from build123d import *

# Parameters (mm, degrees)
SKETCH1_W           = 148
SKETCH1_H           = 62
BOSS_EXTRUDE1_DEPTH = 15
SKETCH2_R           = 2.25
CUT_EXTRUDE1_DEPTH  = 35
SKETCH3_R           = 2.25
CUT_EXTRUDE2_DEPTH  = 25
SKETCH4_W           = 22
SKETCH4_H           = 5
BOSS_EXTRUDE2_DEPTH = 26
SKETCH5_W           = 22
SKETCH5_H           = 5
BOSS_EXTRUDE3_DEPTH = 26
SKETCH6_W           = 20
SKETCH6_H           = 42
BOSS_EXTRUDE4_DEPTH = 15
SKETCH7_W           = 20
SKETCH7_H           = 42
BOSS_EXTRUDE5_DEPTH = 15
SKETCH8_R           = 2.5
CUT_EXTRUDE3_DEPTH  = 25
SKETCH9_R           = 2.5
CUT_EXTRUDE4_DEPTH  = 25
CHAMFER3_SIZE       = 1
CHAMFER4_SIZE       = 1
CHAMFER5_SIZE       = 1
SKETCH10_W          = 27.530750263
SKETCH10_H          = 14.173658936
CUT_EXTRUDE5_DEPTH  = 60
SKETCH11_W          = 32.495188708
SKETCH11_H          = 15.919959855
CUT_EXTRUDE6_DEPTH  = 60
CHAMFER6_SIZE       = 1
CHAMFER7_SIZE       = 1


with BuildPart() as part:
    # Sketch1 → Boss-Extrude1 (new body)
    with BuildSketch(Plane(origin=(0, 0, 0), x_dir=(1, 0, 0), z_dir=(0, 1, 0))):
        with Locations((74, 31)):
            Rectangle(SKETCH1_W, SKETCH1_H)
    extrude(amount=BOSS_EXTRUDE1_DEPTH)

    # Sketch2 → Cut-Extrude1 (cut)
    with BuildSketch(Plane(origin=(0, 15, 0), x_dir=(1, 0, 0), z_dir=(0, 1, 0))):
        with Locations(Location((5, 4, 0), (0, 0, 270))):
            Circle(SKETCH2_R)
        with Locations(Location((20, 4, 0), (0, 0, 270))):
            Circle(SKETCH2_R)
        with Locations(Location((35, 4, 0), (0, 0, 270))):
            Circle(SKETCH2_R)
        with Locations(Location((5, 58, 0), (0, 0, 270))):
            Circle(SKETCH2_R)
        with Locations(Location((20, 58, 0), (0, 0, 270))):
            Circle(SKETCH2_R)
        with Locations(Location((35, 58, 0), (0, 0, 270))):
            Circle(SKETCH2_R)
    extrude(amount=-CUT_EXTRUDE1_DEPTH, mode=Mode.SUBTRACT)

    # Sketch3 → Cut-Extrude2 (cut)
    with BuildSketch(Plane(origin=(0, 15, 0), x_dir=(1, 0, 0), z_dir=(0, 1, 0))):
        with Locations(Location((143, 58, 0), (0, 0, 270))):
            Circle(SKETCH3_R)
        with Locations(Location((143, 4, 0), (0, 0, 270))):
            Circle(SKETCH3_R)
        with Locations(Location((128, 58, 0), (0, 0, 270))):
            Circle(SKETCH3_R)
        with Locations(Location((113, 58, 0), (0, 0, 270))):
            Circle(SKETCH3_R)
        with Locations(Location((128, 4, 0), (0, 0, 270))):
            Circle(SKETCH3_R)
        with Locations(Location((113, 4, 0), (0, 0, 270))):
            Circle(SKETCH3_R)
    extrude(amount=-CUT_EXTRUDE2_DEPTH, mode=Mode.SUBTRACT)

    # Sketch4 → Boss-Extrude2 (add)
    with BuildSketch(Plane(origin=(148, 0, 0), x_dir=(0, 0, -1), z_dir=(1, 0, 0))):
        with Locations((31, 2.5)):
            Rectangle(SKETCH4_W, SKETCH4_H)
    extrude(amount=BOSS_EXTRUDE2_DEPTH)

    # Sketch5 → Boss-Extrude3 (add)
    with BuildSketch(Plane.ZY):
        with Locations((-31, 2.5)):
            Rectangle(SKETCH5_W, SKETCH5_H)
    extrude(amount=BOSS_EXTRUDE3_DEPTH)

    # Sketch6 → Boss-Extrude4 (add)
    with BuildSketch(Plane(origin=(0, 15, 0), x_dir=(1, 0, 0), z_dir=(0, 1, 0))):
        with Locations((184, 31)):
            Rectangle(SKETCH6_W, SKETCH6_H)
    extrude(amount=-BOSS_EXTRUDE4_DEPTH)

    # Sketch7 → Boss-Extrude5 (add)
    with BuildSketch(Plane(origin=(0, 15, 0), x_dir=(1, 0, 0), z_dir=(0, 1, 0))):
        with Locations((-36, 31)):
            Rectangle(SKETCH7_W, SKETCH7_H)
    extrude(amount=-BOSS_EXTRUDE5_DEPTH)

    # Sketch8 → Cut-Extrude3 (cut)
    with BuildSketch(Plane(origin=(0, 15, 0), x_dir=(1, 0, 0), z_dir=(0, 1, 0))):
        with Locations(Location((-36, 46, 0), (0, 0, 270))):
            Circle(SKETCH8_R)
        with Locations(Location((-36, 15, 0), (0, 0, 270))):
            Circle(SKETCH8_R)
    extrude(amount=-CUT_EXTRUDE3_DEPTH, mode=Mode.SUBTRACT)

    # Sketch9 → Cut-Extrude4 (cut)
    with BuildSketch(Plane(origin=(0, 15, 0), x_dir=(1, 0, 0), z_dir=(0, 1, 0))):
        with Locations(Location((184, 46, 0), (0, 0, 270))):
            Circle(SKETCH9_R)
        with Locations(Location((184, 15, 0), (0, 0, 270))):
            Circle(SKETCH9_R)
    extrude(amount=-CUT_EXTRUDE4_DEPTH, mode=Mode.SUBTRACT)

    # Chamfer3
    chamfer3_edges = [part.edges().sort_by_distance(p)[0] for p in [
        (194, 15, -31),
        (-26, 15, -31),
        (-46, 15, -31),
        (161, 5, -20),
    ]]
    chamfer(chamfer3_edges, length=CHAMFER3_SIZE)

    # Chamfer4
    chamfer4_edges = [part.edges().sort_by_distance(p)[0] for p in [
        (-13, 5, -20),
        (-36, 15, -10),
        (-36, 15, -52),
        (183.5, 15, -10),
        (183.5, 15, -52),
        (161, 5, -42),
    ]]
    chamfer(chamfer4_edges, length=CHAMFER4_SIZE)

    # Chamfer5
    chamfer5_edges = [part.edges().sort_by_distance(p)[0] for p in [
        (-13, 5, -42),
        (174, 15, -31),
    ]]
    chamfer(chamfer5_edges, length=CHAMFER5_SIZE)

    # Sketch10 → Cut-Extrude5 (cut)
    with BuildSketch(Plane(origin=(0, 0, -52), x_dir=(-1, 0, 0), z_dir=(0, 0, -1))):
        with Locations((-183.765375132, 12.086829468)):
            Rectangle(SKETCH10_W, SKETCH10_H)
    extrude(amount=-CUT_EXTRUDE5_DEPTH, mode=Mode.SUBTRACT)

    # Sketch11 → Cut-Extrude6 (cut)
    with BuildSketch(Plane(origin=(0, 0, -52), x_dir=(-1, 0, 0), z_dir=(0, 0, -1))):
        with Locations((37.724079719, 12.959979928)):
            Rectangle(SKETCH11_W, SKETCH11_H)
    extrude(amount=-CUT_EXTRUDE6_DEPTH, mode=Mode.SUBTRACT)

    # Chamfer6
    chamfer6_edges = [part.edges().sort_by_distance(p)[0] for p in [
        (174, 5, -46.5),
        (194, 5, -31),
        (174, 5, -15.5),
        (-46, 5, -31),
        (-36, 5, -10),
        (-26, 5, -46.5),
    ]]
    chamfer(chamfer6_edges, length=CHAMFER6_SIZE)

    # Chamfer7
    chamfer7_edges = [part.edges().sort_by_distance(p)[0] for p in [
        (-36, 5, -52),
        (-26, 5, -16),
        (184, 5, -10),
        (184, 5, -52),
    ]]
    chamfer(chamfer7_edges, length=CHAMFER7_SIZE)


solid = part.part
Verification items for the finished model (mm, model axes). A direction names the side the tool comes from. Give positions to 0.01 mm unless a question says otherwise; leave off trailing zeros. Write each loop counter-clockwise with the first axis right and the second up, starting at its lowest first coordinate (ties: lowest second). Pieces come first, ordered by that corner, then holes.
(1) Material ranges on line 1 (Z direction, x = 143, y = 11); line 2 (X direction, y = 2.3, z = -15); line 3 (Z direction, x = 19, y = 1.5), recorded low to high.
(2) Cross-section at B-B (z = -46). Enter the section's corners in (x, y), plus the area to 3 significant figures.
(3) Mould release check, pull along Z, two halves, no side actions. Record for faces 1 (the face through (174, 2, -15)), 2 (the face through (37.23, 7.6, -4.29)), 3 (the face through (184, 2, -10)): +Z half, -Z half, draft (parallel to the pull), parting line (faces both ways), or undercut.
(4) Gauge pin test, flat ends, axial feed: pin 1 (4 mm diameter, centred on x = 5, z = -58, fed in from +Y); pin 2 (4.5 mm diameter, centred on x = -19.5, y = 2.5, fed in from -Z); pin 3 (6.5 mm diameter, centred on x = 184, z = -46, fed in from +Y); pin 4 (3 mm diameter, centred on y = 7, z = -49, fed in from +X). Record the tip position at first contact, or that the pin passes through.
(5) Cross-section at A-A (x = 128). Enter the section's corners in (y, z), plus the area to 3 significant figures.
(6) Cross-section at D-D (y = 10). State how many separate pieces and enclosed holes the cut face has, plus the area to 3 significant figures.
(7) Cross-section at C-C (z = -4). Enter the section's corners in (x, y).
(8) Access from +Z, -Z, +X, -X, +Y, -Y to the whole of each face (thin tool, end or side, straight path). Record for faces 4 (the face through (-13, 2, -42)), 5 (the face through (-27, 5, -31)), 6 (the face through (-26, 2, -15)).
Worked out:
1. line 1: z = -62 to -60.25, -55.75 to -6.25, -1.75 to 0
1. line 2: x = -46 to -38.5, -33.5 to -26, 0 to 148, 174 to 181.5, 186.5 to 194
1. line 3: z = -62 to -60.02, -55.98 to -6.02, -1.98 to 0
2. outline: (-46, 0) - (-38.5, 0) - (-38.5, 5) - (-45, 5) - (-46, 4) - close; (-33.5, 0) - (-26, 0) - (-26, 4) - (-27, 5) - (-33.5, 5) - close; (0, 0) - (148, 0) - (148, 15) - (0, 15) - close; (174, 0) - (181.5, 0) - (181.5, 5) - (175, 5) - (174, 4) - close; (186.5, 0) - (194, 0) - (194, 4) - (193, 5) - (186.5, 5) - close
2. area: 2,370 mm2
3. face 1: draft
3. face 2: undercut
3. face 3: +Z half
4. pin 1: passes through
4. pin 2: stops at z = -42
4. pin 3: stops at y = 5
4. pin 4: stops at x = 148
5. outline: (0, -62) - (15, -62) - (15, -60.25) - (0, -60.25) - close; (0, -55.75) - (15, -55.75) - (15, -6.25) - (0, -6.25) - close; (0, -1.75) - (15, -1.75) - (15, 0) - (0, 0) - close
5. area: 795 mm2
6. separate pieces: 1
6. enclosed holes: 12
6. area: 8,990 mm2
7. outline: (0, 0) - (2.75, 0) - (2.75, 15) - (0, 15) - close; (7.25, 0) - (17.75, 0) - (17.75, 15) - (7.25, 15) - close; (22.25, 0) - (32.75, 0) - (32.75, 15) - (22.25, 15) - close; (37.25, 0) - (110.75, 0) - (110.75, 15) - (37.25, 15) - close; (115.25, 0) - (125.75, 0) - (125.75, 15) - (115.25, 15) - close; (130.25, 0) - (140.75, 0) - (140.75, 15) - (130.25, 15) - close; (145.25, 0) - (148, 0) - (148, 15) - (145.25, 15) - close
8. face 4: -Z, +Y, -Y
8. face 5: +Z, -Z, -X, +Y
8. face 6: +Z, +Y, -Y
